```python
from build123d import *

# Parameters (mm, degrees)
SKETCH1_R               = 7.5
BOSS_EXTRUDE1_DEPTH     = 24
SKETCH2_R               = 4
CUT_EXTRUDE1_DEPTH      = 5
CUT_EXTRUDE2_DEPTH      = 56.410648796
CUT_EXTRUDE2_DEPTH_BACK = 56.410648796
BOSS_EXTRUDE2_START     = 5.5
SKETCH4_W               = 38
SKETCH4_H               = 15
SKETCH4_R               = 4
BOSS_EXTRUDE2_DEPTH     = 5.5
CUT_EXTRUDE3_DEPTH      = 56.410648965
CUT_EXTRUDE3_DEPTH_BACK = 56.410648965
SKETCH5_R               = 1.875
SKETCH6_R               = 1.85
CUT_EXTRUDE4_DEPTH      = 9


with BuildPart() as part:
    # Sketch1 → Boss-Extrude1 (new, symmetric)
    with BuildSketch(Plane.XY):
        with BuildLine():
            Line((-17.47471084, 5.003045957), (-16.099481109, 12.802361333))
            ThreePointArc((-16.099481109, 12.802361333), (-13.534330034, 17.245333323), (-8.713422961, 19))
            Line((-8.713422961, 19), (7.5, 19))
            ThreePointArc((7.5, 19), (13.863961031, 16.363961031), (16.5, 10))
            Line((16.5, 10), (25, 10))
            Line((25, 10), (25, 25))
            Line((25, 25), (12.627503281, 25))
            Line((12.627503281, 25), (-40.3, 25))
            Line((-40.3, 25), (-40.3, 7))
            ThreePointArc((-40.3, 7), (-29.802291042, -4.456239028), (-17.47471084, 5.003045957))
        make_face()
        with Locations((-28.8, 7)):
            Circle(SKETCH1_R, mode=Mode.SUBTRACT)
    extrude(amount=BOSS_EXTRUDE1_DEPTH, both=True)

    # Sketch2 → Cut-Extrude1 (cut)
    with BuildSketch(Plane(origin=(25, 0, 0), x_dir=(0, 0, -1), z_dir=(1, 0, 0))):
        with Locations((-12.5, 17)):
            Circle(SKETCH2_R)
        with Locations((12.5, 17)):
            Circle(SKETCH2_R)
    extrude(amount=-CUT_EXTRUDE1_DEPTH, mode=Mode.SUBTRACT)

    # Sketch3 → Cut-Extrude2 (cut, two sides: drawn at the far end of the back side and taken through both)
    with BuildSketch(Plane(origin=(0, 25, 0), x_dir=(1, 0, 0), z_dir=(0, 1, 0)).offset(-CUT_EXTRUDE2_DEPTH_BACK)):
        with BuildLine():
            Line((-28.8, -24), (25, -24))
            Line((25, -24), (25, -19))
            Line((25, -19), (21, -19))
            ThreePointArc((21, -19), (17.364289008, -18.552718151), (13.94540302, -17.237547411))
            ThreePointArc((13.94540302, -17.237547411), (-3.160771505, -13.862715808), (-19.25459698, -20.570880744))
            ThreePointArc((-19.25459698, -20.570880744), (-23.728669364, -23.116713696), (-28.8, -24))
        make_face()
        with BuildLine():
            Line((21, 19), (25, 19))
            Line((25, 19), (25, 24))
            Line((25, 24), (-28.8, 24))
            ThreePointArc((-28.8, 24), (-23.728669364, 23.116713696), (-19.25459698, 20.570880744))
            ThreePointArc((-19.25459698, 20.570880744), (-3.160771505, 13.862715808), (13.94540302, 17.237547411))
            ThreePointArc((13.94540302, 17.237547411), (17.364289008, 18.552718151), (21, 19))
        make_face()
    extrude(amount=CUT_EXTRUDE2_DEPTH + CUT_EXTRUDE2_DEPTH_BACK, mode=Mode.SUBTRACT)

    # Sketch4 → Boss-Extrude2 (add)
    with BuildSketch(Plane(origin=(25, 0, 0), x_dir=(0, 0, -1), z_dir=(1, 0, 0)).offset(BOSS_EXTRUDE2_START)):
        with Locations((0, 17.5)):
            Rectangle(SKETCH4_W, SKETCH4_H)
        with Locations((12.5, 17)):
            Circle(SKETCH4_R, mode=Mode.SUBTRACT)
        with Locations((-12.5, 17)):
            Circle(SKETCH4_R, mode=Mode.SUBTRACT)
    extrude(amount=-BOSS_EXTRUDE2_DEPTH)

    # Sketch5 → Cut-Extrude3 (cut, two sides: drawn at the far end of the back side and taken through both)
    with BuildSketch(Plane(origin=(0, 25, 0), x_dir=(1, 0, 0), z_dir=(0, 1, 0)).offset(-CUT_EXTRUDE3_DEPTH_BACK)):
        with Locations(Location((25.5, -5, 0), (0, 0, 180))):
            Circle(SKETCH5_R)
        with Locations(Location((25.5, 5, 0), (0, 0, 180))):
            Circle(SKETCH5_R)
    extrude(amount=CUT_EXTRUDE3_DEPTH + CUT_EXTRUDE3_DEPTH_BACK, mode=Mode.SUBTRACT)

    # Sketch6 → Cut-Extrude4 (cut)
    with BuildSketch(Plane(origin=(0, 25, 0), x_dir=(1, 0, 0), z_dir=(0, 1, 0))):
        with Locations(Location((-28.8, 16, 0), (0, 0, 270))):
            Circle(SKETCH6_R)
        with Locations(Location((-28.8, 0, 0), (0, 0, 270))):
            Circle(SKETCH6_R)
        with Locations(Location((-28.8, -16, 0), (0, 0, 270))):
            Circle(SKETCH6_R)
    extrude(amount=-CUT_EXTRUDE4_DEPTH, mode=Mode.SUBTRACT)


solid = part.part
```
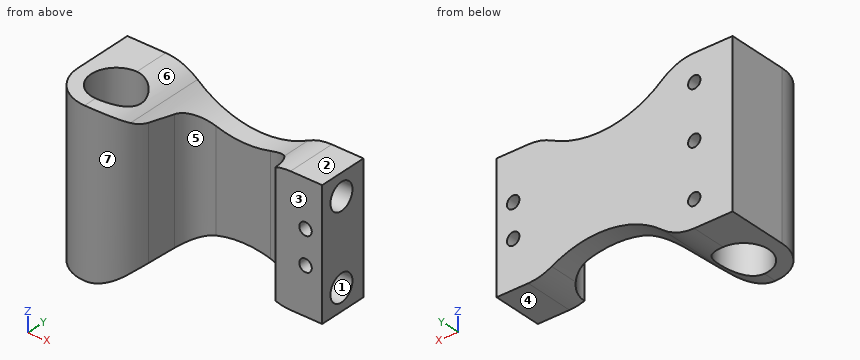
The model under review builds one solid part; all positions refer to its coordinate system, in mm. Face numbers are marked on the shaded views. A direction names the side the tool comes from. Coordinates: 2 decimals unless noted, no trailing zeros. Order: outer loops, then holes, each group sorted by start corner. A loop starts at its lowest first (then second) coordinate and runs counter-clockwise, first axis right, second up. Notation, with made-up numbers: (5, 12) -> (12, 12) arc R27 ccw to (12, 39) -> close; hole circle Ø10 at (-37, 7). An arc over 180 degrees is marked (long way). Answer in a Markdown table with one row per item. Add a question column.
Item 1: Clearance check with flat-ended pins moving along their axes: pin 1 (1 mm diameter, centred on y = 9, z = -10, fed in from +X); pin 2 (12 mm diameter, centred on x = 11, z = -4.5, fed in from -Y); pin 3 (7 mm diameter, centred on y = 17, z = -12.5, fed in from +X); pin 4 (9 mm diameter, centred on x = -28.8, y = 7, fed in from +Z). State where each tip first meets the part, or that it passes through.
Item 2: We need section A-A on z = 5. Write out the cut boundary in (x, y) (3 decimals).
Item 3: To check wall thickness, follow probe 1 along Z at (x, y) = (25.5, 12.5) (3 decimals); probe 2 along X at (y, z) = (13.5, -6); probe 3 along Z at (x, y) = (25.5, 18) (3 decimals). State the ranges of each line that lie inside material, in increasing order.
Item 4: Mouldability with a two-part tool opening along X and no side actions: class the marked faces 5, 6 and 7 as +X half, -X half, draft (parallel to the pull), parting line (faces both ways), or undercut.
Item 5: Machinability: for the marked faces 1, 2, 3 and 4, which of the approach directions +Z, -Z, +X, -X, +Y, -Y give a long, thin tool a straight path to every point of the face, cutting with its end or side? Answer none if there is none.
Item 6: We need section C-C on y = 6. Write out the cut boundary in (x, z), plus the area to 3 significant figures.
Item 7: We need section B-B on z = 12.5. Write out the cut boundary in (x, y), plus the area to 3 significant figures.
Item 8: We need section D-D on x = -7.5. Write out the cut boundary in (y, z), plus the area to 3 significant figures.
Final values:
| question | item | result |
|---|---|---|
| 1 | pin 1 | stops at x = -16.68 |
| 1 | pin 2 | stops at y = 10 |
| 1 | pin 3 | stops at x = 20 |
| 1 | pin 4 | passes through |
| 2 | outline | (-40.3, 7) arc R11.5 ccw to (-17.475, 5.003) -> (-16.099, 12.802) arc R7.5 cw to (-8.713, 19) -> (7.5, 19) arc R9 cw to (16.5, 10) -> (23.625, 10) -> (23.625, 25) -> (-40.3, 25) -> close; (27.375, 10) -> (30.5, 10) -> (30.5, 25) -> (27.375, 25) -> close; hole circle Ø15 at (-28.8, 7) |
| 3 | probe 1 | z = -19 to -6.875, -3.125 to 3.125, 6.875 to 19 |
| 3 | probe 2 | x = -40.3 to -32.54, -25.06 to -15.94, 15.79 to 23.91, 27.09 to 30.5 |
| 3 | probe 3 | z = -19 to -16.373, -8.627 to -6.875, -3.125 to 3.125, 6.875 to 8.627, 16.373 to 19 |
| 4 | face 5 | undercut |
| 4 | face 6 | +X half |
| 4 | face 7 | parting line |
| 5 | face 1 | +X |
| 5 | face 2 | +Z, +X, +Y, -Y |
| 5 | face 3 | +Z, -Z, +X, -Y |
| 5 | face 4 | -Z, +X, +Y, -Y |
| 6 | outline | (-40.26, -24) -> (-36.23, -24) -> (-36.23, 24) -> (-40.26, 24) -> close; (-21.37, -22.03) arc R15 ccw to (-19.25, -20.57) arc R30 cw to (-17.3, -19.09) -> (-17.3, 19.09) arc R30 cw to (-19.25, 20.57) arc R15 ccw to (-21.37, 22.03) -> close |
| 6 | area | 361 mm2 |
| 7 | outline | (-40.3, 7) arc R11.5 ccw to (-17.47, 5) -> (-16.1, 12.8) arc R7.5 cw to (-8.71, 19) -> (7.5, 19) arc R9 cw to (16.5, 10) -> (30.5, 10) -> (30.5, 13) -> (20, 13) -> (20, 21) -> (30.5, 21) -> (30.5, 25) -> (-40.3, 25) -> close; hole circle Ø15 at (-28.8, 7) |
| 7 | area | 814 mm2 |
| 8 | outline | (19, -14.62) -> (25, -14.62) -> (25, 14.62) -> (19, 14.62) -> close |
| 8 | area | 175 mm2 |
